from build123d import *

# Parameters (mm, degrees)
ESQUISSE1_W                                        = 200
ESQUISSE1_H                                        = 200
BOSS_EXTRU_1_DEPTH                                 = 10
ESQUISSE2_R                                        = 15
ENL_V_MAT_EXTRU_1_DEPTH                            = 142.774468788
CHANFREIN1_SIZE                                    = 3
CHAMBRAGE_POUR_VIS_T_TE_HEXAGONALE_M41_D           = 4.5
CHAMBRAGE_POUR_VIS_T_TE_HEXAGONALE_M41_CBORE_D     = 8
CHAMBRAGE_POUR_VIS_T_TE_HEXAGONALE_M41_CBORE_DEPTH = 4.4
TROUS_DE_CENTRAGE_4_0MMCLEARANCE_1_D               = 4
CHAMBRAGE_POUR_VIS_T_TE_HEXAGONALE_M61_D           = 6.6
CHAMBRAGE_POUR_VIS_T_TE_HEXAGONALE_M61_CBORE_D     = 11
CHAMBRAGE_POUR_VIS_T_TE_HEXAGONALE_M61_CBORE_DEPTH = 7.4
TROU_TARAUD_M41_D                                  = 3.3
TROU_TARAUD_M41_DEPTH                              = 14
TROU_TARAUD_M41_TIP                                = 0.991420021
TROU_TARAUD_M42_D                                  = 3.3
TROU_TARAUD_M42_DEPTH                              = 14
TROU_TARAUD_M42_TIP                                = 0.991420021
TROU_TARAUD_M52_D                                  = 4.2
TROU_TARAUD_M52_DEPTH                              = 15


with BuildPart() as part:
    # Esquisse1 → Boss.-Extru.1 (new body)
    with BuildSketch(Plane.XY):
        Rectangle(ESQUISSE1_W, ESQUISSE1_H)
    extrude(amount=BOSS_EXTRU_1_DEPTH)

    # Esquisse2 → Enlèv. mat.-Extru.1 (cut, through all)
    with BuildSketch(Plane.XY.offset(10)):
        with Locations((-9.5, 0)):
            Circle(ESQUISSE2_R)
    extrude(amount=-ENL_V_MAT_EXTRU_1_DEPTH, mode=Mode.SUBTRACT)

    # Chanfrein1
    chanfrein1_edges = [part.edges().sort_by_distance(p)[0] for p in [
        (-100, 100, 5),
        (100, 100, 5),
        (100, -100, 5),
        (-100, -100, 5),
    ]]
    chamfer(chanfrein1_edges, length=CHANFREIN1_SIZE)

    # Chambrage pour vis à tête hexagonale M41 (through all)
    with Locations(Plane(origin=(54.5, 32.7, 10), x_dir=(1, 0, 0), z_dir=(0, 0, 1))):
        with Locations((0, 0), (0, -64)):
            CounterBoreHole(CHAMBRAGE_POUR_VIS_T_TE_HEXAGONALE_M41_D / 2, CHAMBRAGE_POUR_VIS_T_TE_HEXAGONALE_M41_CBORE_D / 2, CHAMBRAGE_POUR_VIS_T_TE_HEXAGONALE_M41_CBORE_DEPTH)

    # Trous de centrage Ø4.0mmClearance 1 (through all)
    with Locations(Plane(origin=(54.5, -18.3, 10), x_dir=(1, 0, 0), z_dir=(0, 0, 1))):
        with Locations((0, 0), (0, 38)):
            Hole(TROUS_DE_CENTRAGE_4_0MMCLEARANCE_1_D / 2)

    # Chambrage pour vis à tête hexagonale M61 (through all)
    with Locations(Plane.XY.offset(10)):
        with Locations((23, 0), (-9.5, 32.5), (-42, 0), (-9.5, -32.5)):
            CounterBoreHole(CHAMBRAGE_POUR_VIS_T_TE_HEXAGONALE_M61_D / 2, CHAMBRAGE_POUR_VIS_T_TE_HEXAGONALE_M61_CBORE_D / 2, CHAMBRAGE_POUR_VIS_T_TE_HEXAGONALE_M61_CBORE_DEPTH)

    # Trou taraudé M41
    with Locations(Plane(origin=(0, 100, 0), x_dir=(1, 0, 0), z_dir=(0, 1, 0))):
        with Locations((-75, -5), (0, -5), (75, -5)):
            Hole(TROU_TARAUD_M41_D / 2, depth=TROU_TARAUD_M41_DEPTH)
            with Locations((0, 0, -(TROU_TARAUD_M41_DEPTH + TROU_TARAUD_M41_TIP / 2))):  # 118° drill point
                Cone(0, TROU_TARAUD_M41_D / 2, TROU_TARAUD_M41_TIP, mode=Mode.SUBTRACT)

    # Trou taraudé M42
    with Locations(Plane(origin=(0, -100, 0), x_dir=(-1, 0, 0), z_dir=(0, -1, 0))):
        with Locations((75, -5), (0, -5), (-75, -5)):
            Hole(TROU_TARAUD_M42_D / 2, depth=TROU_TARAUD_M42_DEPTH)
            with Locations((0, 0, -(TROU_TARAUD_M42_DEPTH + TROU_TARAUD_M42_TIP / 2))):  # 118° drill point
                Cone(0, TROU_TARAUD_M42_D / 2, TROU_TARAUD_M42_TIP, mode=Mode.SUBTRACT)

    # Trou taraudé M52
    with Locations(Plane.ZY.offset(100)):
        with Locations((5, 0), (5, -75), (5, 75)):
            Hole(TROU_TARAUD_M52_D / 2, depth=TROU_TARAUD_M52_DEPTH)


solid = part.part
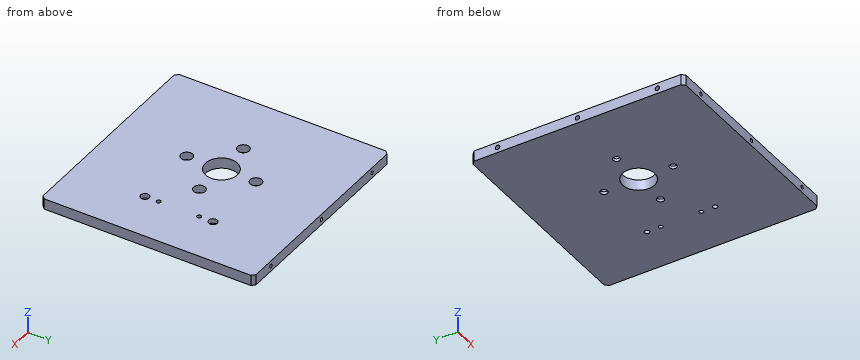
For this review, take the finished solid that the model builds, in its own axes (mm). Round coordinates to 2 decimals unless told otherwise and drop trailing zeros. Write each loop counter-clockwise with the first axis right and the second up, starting at its lowest first coordinate (ties: lowest second). Pieces come first, ordered by that corner, then holes. Notation, with made-up numbers: (42.25, 23.25) -> (101.25, 23.25) arc R26 ccw to (101.25, 43.25) -> close; hole circle Ø3 at (-29, 44). An arc over 180 degrees is marked (long way). Put each result on its own line as item: value.
Q1. To check wall thickness, follow L1, parallel to X at y = -89.5, z = 5; L2, parallel to Y at x = -9.5, z = 6.75; L3, parallel to Z at x = 75, y = -95.75. State the ranges of each line that lie inside material, in increasing order. Write a range as [from, to].
Determined:
L1: x = [-100, -76.65], [-73.35, -1.65], [1.65, 73.35], [76.65, 100]
L2: y = [-100, -38], [-27, -15], [15, 27], [38, 100]
L3: z = [0, 3.35], [6.65, 10]
Q2. Consider section B-B on x = -9.5. State the section outline as (y, z) points.
Determined:
outline: (-100, 0) -> (-35.8, 0) -> (-35.8, 2.6) -> (-38, 2.6) -> (-38, 10) -> (-100, 10) -> close; (-29.2, 0) -> (-15, 0) -> (-15, 10) -> (-27, 10) -> (-27, 2.6) -> (-29.2, 2.6) -> close; (15, 0) -> (29.2, 0) -> (29.2, 2.6) -> (27, 2.6) -> (27, 10) -> (15, 10) -> close; (35.8, 0) -> (100, 0) -> (100, 10) -> (38, 10) -> (38, 2.6) -> (35.8, 2.6) -> close
Q3. Clearance check with flat-ended pins moving along their axes: pin 1 Ø10.5 at (x, y) = (23, 0) entering from +Z; pin 2 Ø7 at (x, y) = (54.5, 32.7) entering from +Z; pin 3 Ø3 at (x, z) = (-75, 5) entering from -Y; pin 4 Ø4 at (x, y) = (-9.5, -32.5) entering from +Z. State where each tip first meets the part, or that it passes through.
Determined:
pin 1: stops at z = 2.6
pin 2: stops at z = 5.6
pin 3: stops at y = -85.91
pin 4: passes through
Q4. Consider section A-A on x = -42. State the section outline as (y, z) points.
Determined:
outline: (-100, 0) -> (-3.3, 0) -> (-3.3, 2.6) -> (-5.5, 2.6) -> (-5.5, 10) -> (-100, 10) -> close; (3.3, 0) -> (100, 0) -> (100, 10) -> (5.5, 10) -> (5.5, 2.6) -> (3.3, 2.6) -> close
